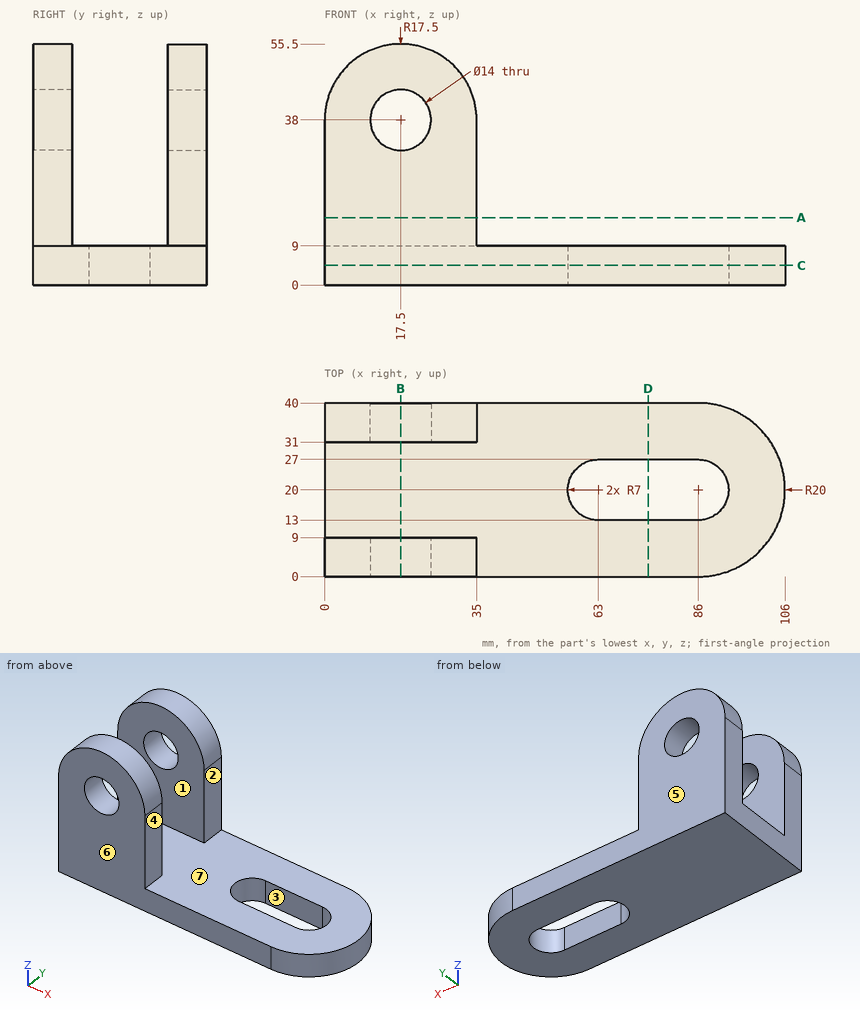
The figure shows three views and two pictorial views of one solid part (mm, origin at its lowest corner). Answer the questions. A direction names the side the tool comes from. Round coordinates to 2 decimals unless told otherwise and drop trailing zeros. Loops run counter-clockwise (first coordinate to the right, second up) from the corner with the lowest first, then second, coordinate; pieces in that order, holes last. Notation, with made-up numbers: M 79,82.25 L 123,82.25 A25 ccw 123,105.25 Z; hole C 75.25,-37.5 d8. An arc over 180 degrees is marked long. Write each question's results on one line, items separated by ' | '. Start each with the question number.
1) Find section D-D on x = 74.5. Write down the section's boundary in (y, z).
2) Find section B-B on x = 17.5. Write down the section's boundary in (y, z).
3) Each of these flat-tipped pins is pushed along its axis until it touches: pin 1 (3 mm diameter, centred on y = 22.5, z = 6.5, fed in from -X); pin 2 (1 mm diameter, centred on x = 19.5, y = 10, fed in from +Z); pin 3 (8.5 mm diameter, centred on x = 17.5, z = 38, fed in from -Y); pin 4 (10 mm diameter, centred on y = 5, z = 30, fed in from +X). Where does it stop, or does it pass through?
4) Determine the mould class of the marked faces 4, 5, 6 and 7 for opening direction Y: pulls with the +Y half, pulls with the -Y half, needs draft (parallel to the pull), parting line crosses it, or undercut.
5) Find section A-A on z = 15.5. Write down the section's boundary in (x, y).
6) Which of the six approach directions +Z, -Z, +X, -X, +Y, -Y give full straight-line access (tool end or side, diameter ignored) to the marked faces 1, 2 and 3?
7) Find section C-C on z = 4.5. Write down the section's boundary in (x, y), plus the area to 3 significant figures.
8) Straight lines are drawn through the part: probe 1 along Y at (x, z) = (5, 22); probe 2 along Z at (x, y) = (17, 4); probe 3 along X at (y, z) = (2, 14.5). For each, find the intervals that lie inside material, in ascending order.
Final values:
1) outline: M 0,0 L 13,0 L 13,9 L 0,9 Z; M 27,0 L 40,0 L 40,9 L 27,9 Z
2) outline: M 0,0 L 40,0 L 40,31 L 31,31 L 31,9 L 9,9 L 9,31 L 0,31 Z; M 0,45 L 9,45 L 9,55.5 L 0,55.5 Z; M 31,45 L 40,45 L 40,55.5 L 31,55.5 Z
3) pin 1: x = 0 | pin 2: z = 9 | pin 3: through | pin 4: x = 35
4) face 4: needs draft | face 5: pulls with the +Y half | face 6: pulls with the -Y half | face 7: undercut
5) outline: M 0,0 L 35,0 L 35,9 L 0,9 Z; M 0,31 L 35,31 L 35,40 L 0,40 Z
6) face 1: +Z, +X, -X | face 2: +Z, +X, +Y, -Y | face 3: +Z, -Z
7) outline: M 0,0 L 86,0 A20 ccw 86,40 L 0,40 Z; hole M 63,13 L 86,13 A7 ccw 86,27 L 63,27 A7 ccw Z | area: 3,590 mm²
8) probe 1: 0 to 9, 31 to 40 | probe 2: 0 to 31.02, 44.98 to 55.49 | probe 3: 0 to 35
